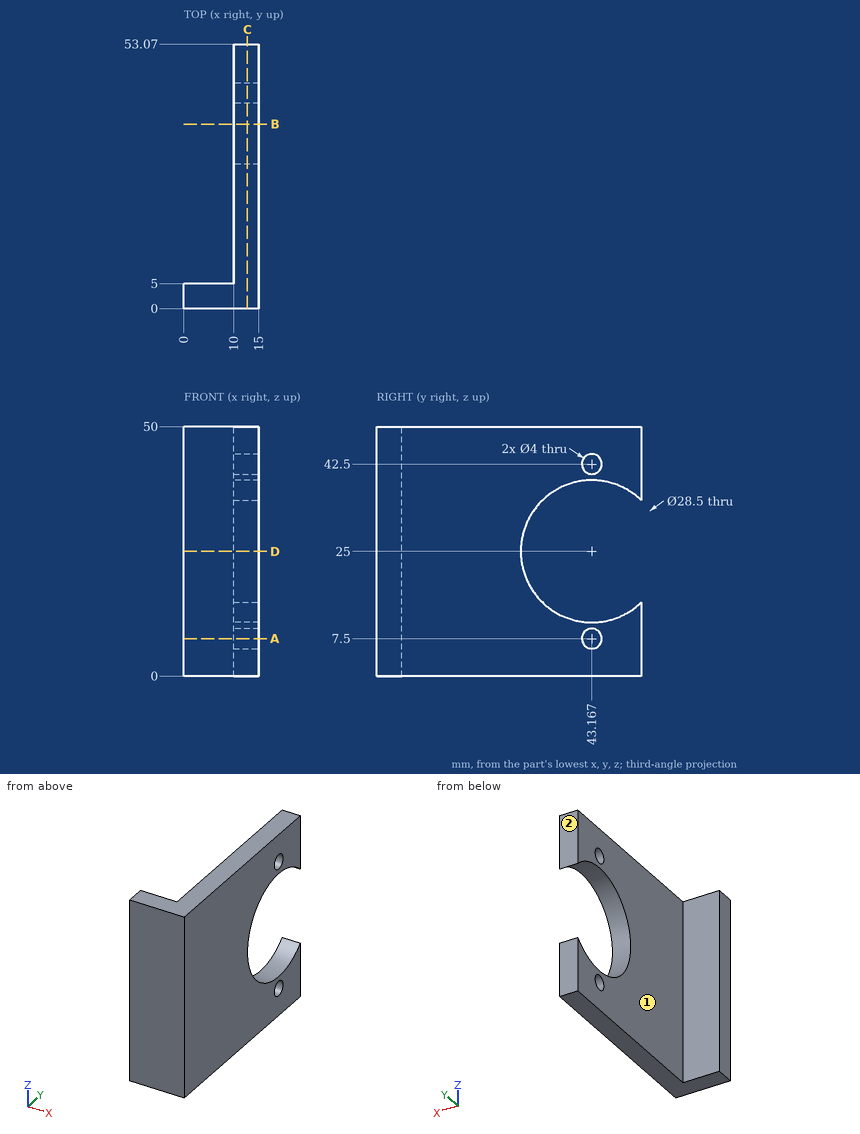
For this review, use the dimensioned drawing (mm, ordinates from the lowest corner) and the shaded views. A direction names the side the tool comes from. Round coordinates to 2 decimals unless told otherwise and drop trailing zeros. Order: outer loops, then holes, each group sorted by start corner. A loop starts at its lowest first (then second) coordinate and runs counter-clockwise, first axis right, second up. Notation, with made-up numbers: (77, 70.25) - (118, 70.25) arc R17 ccw to (118, 76.25) - close; hole circle Ø6 at (-31, 53). An arc over 180 degrees is marked (long way). Use one line per item in the form item = value.
Q1. To check wall thickness, follow line 1 (Y direction, x = 13.15, z = 7.5); line 2 (Z direction, x = 13.5, y = 42); line 3 (X direction, y = 11, z = 26). State the ranges of each line that lie inside material, in increasing order.
Response values:
line_1 = 0 to 41.17, 45.17 to 53.07
line_2 = 0 to 5.88, 9.12 to 10.8, 39.2 to 40.88, 44.12 to 50
line_3 = 10 to 15
Q2. Add section A-A on z = 7.5. Give the boundary of the cut face in (x, y), then the cut area to 3 significant figures.
Response values:
outline = (0, 0) - (15, 0) - (15, 41.17) - (10, 41.17) - (10, 5) - (0, 5) - close; (10, 45.17) - (15, 45.17) - (15, 53.07) - (10, 53.07) - close
area = 295 mm^2
Q3. Tool access review of the marked faces 1 and 2: name each direction out of +Z, -Z, +X, -X, +Y, -Y from which nothing blocks a thin tool from reaching the whole face with its end or side.
Response values:
face_1 = +Z, -Z, -X, +Y
face_2 = +Z, -Z, +X, -X, +Y
Q4. Add section B-B on y = 37. Give the boundary of the cut face in (x, z).
Response values:
outline = (10, 0) - (15, 0) - (15, 12.15) - (10, 12.15) - close; (10, 37.85) - (15, 37.85) - (15, 50) - (10, 50) - close
Q5. Add section C-C on x = 12.75. Give the boundary of the cut face in (y, z).
Response values:
outline = (0, 0) - (53.07, 0) - (53.07, 14.75) arc R14.25 cw (long way) to (53.07, 35.25) - (53.07, 50) - (0, 50) - close; hole circle Ø4 at (43.17, 7.5); hole circle Ø4 at (43.17, 42.5)
Q6. Add section D-D on z = 25. Give the boundary of the cut face in (x, y).
Response values:
outline = (0, 0) - (15, 0) - (15, 28.92) - (10, 28.92) - (10, 5) - (0, 5) - close
Q7. Clearance check with flat-ended pins moving along their axes: P1, Ø1.5, axis at x = 7, z = 10.5, coming from the +Y side; P2, Ø1, axis at y = 11, z = 9.5, coming from the -X side; P3, Ø3.5, axis at y = 43.17, z = 7.5, coming from the +X side. State where each tip first meets the part, or that it passes through.
Response values:
P1 = 5
P2 = 10
P3 = through
